Build history of the part. All positions in model axes, mm. A direction names the side the tool comes from. Round coordinates to 2 decimals unless told otherwise and drop trailing zeros. Loops run counter-clockwise (first coordinate to the right, second up) from the corner with the lowest first, then second, coordinate; pieces in that order, holes last. Notation, with made-up numbers: M 70,56.25 L 80,56.25 A7 ccw 80,69.25 Z; hole C 1,-23.75 d4. An arc over 180 degrees is marked long. One line per item, written item: value.
```python
from build123d import *

# Parameters (mm, degrees)
F0_W     = 101.6
F0_H     = 25.4
F1_DEPTH = 76.2
F3_DEPTH = 25.4
F5_DEPTH = 25.4


with BuildPart() as f1:
    # F0 (on Front) → F1 (new body)
    with BuildSketch(Plane.XZ):
        with Locations((-4.908444, -38.063884)):
            Rectangle(F0_W, F0_H)
    extrude(amount=F1_DEPTH)

    # F2 (on face) → F3 (join)
    with BuildSketch(Plane.XY.offset(-25.363884)):
        Polygon((20.491556, -76.2), (45.891556, -76.2), (45.891556, -38.1), align=None)
    extrude(amount=F3_DEPTH)

    # F4 (on face) → F5 (join)
    with BuildSketch(Plane.XY.offset(-25.363884)):
        Polygon((-55.708444, 0), (-55.708444, -76.2), (-43.008444, -76.2), (20.491556, 0), align=None)
    extrude(amount=F5_DEPTH)


solid = f1.part
```
Item 1: Slice it at B-B, the plane y = -25.5. Give the cut face in (x, z).
Check values:
outline: M -55.71,-50.76 L 45.89,-50.76 L 45.89,-25.36 L -0.76,-25.36 L -0.76,0.04 L -55.71,0.04 Z
Item 2: Which spindle directions (+Z, -Z, +X, -X, +Y, -Y) get a long thin tool onto all of the face, cutting with end or side? Do faces 5 (the face through (-6, -76.2, -31)), 6 (the face through (33.37, -56.88, -12.84)). Say none if no direction does.
Check values:
face 5: +Z, -Z, +X, -X, -Y
face 6: +Z, +Y
Item 3: Slice it at D-D, the plane y = -63.5. Give the cut face in (x, z).
Check values:
outline: M -55.71,-50.76 L 45.89,-50.76 L 45.89,0.04 L 28.96,0.04 L 28.96,-25.36 L -32.43,-25.36 L -32.43,0.04 L -55.71,0.04 Z
Item 4: Pull direction X, two halves, no side cores. Call faces 1 (the face through (39, -65, 0.036)), 2 (the face through (-11.7, -38.63, -12.84)), 3 (the face through (11, -46, -25.364)), 4 (the face through (45.892, -47, -31)): pulls with the +X half, pulls with the -X half, needs draft (parallel to the pull), parting line crosses it, or undercut.
Check values:
face 1: needs draft
face 2: undercut
face 3: undercut
face 4: pulls with the +X half
Item 5: Slice it at A-A, the plane z = -14.5. Give the cut face in (x, y), and give its area (3 significant figures).
Check values:
outline: M -55.71,-76.2 L -43.01,-76.2 L 20.49,0 L -55.71,0 Z; M 20.49,-76.2 L 45.89,-76.2 L 45.89,-38.1 Z
area: 3,870 mm2
Item 6: Slice it at C-C, the plane x = -21.5. Give the cut face in (y, z).
Check values:
outline: M -76.2,-50.76 L 0,-50.76 L 0,0.04 L -50.39,0.04 L -50.39,-25.36 L -76.2,-25.36 Z
Item 7: Drop flat-ended pins along their axis: P1, Ø3, axis at x = -13.5, z = -40, coming from the +Y side; P2, Ø1, axis at x = -10.5, y = -43, coming from the +Z side. Give the stop position or say it passes through.
Check values:
P1: stops at y = 0
P2: stops at z = -25.36
Item 8: Wall check: line 1 along Z through (x, y) = (30, -45); line 2 along Y through (x, z) = (-28, -9.5); line 3 along X through (y, z) = (-72, -21). Give the ranges that are in metal, low to high.
Check values:
line 1: z = -50.76 to -25.36
line 2: y = -58.19 to 0
line 3: x = -55.71 to -39.51, 23.29 to 45.89
